Could you check a few things on this model? Use its own coordinates, in mm. A direction names the side the tool comes from. Coordinates: 2 decimals unless noted, no trailing zeros. Loops run counter-clockwise (first coordinate to the right, second up) from the corner with the lowest first, then second, coordinate; pieces in that order, holes last. Notation, with made-up numbers: (-4.5, -18.75) - (26.5, -18.75) arc R19 cw to (26.5, 0.25) - close; hole circle Ø4 at (43, 52). An arc over 180 degrees is marked (long way). One line per question, with ' | ' between items. Start each with the question number.
1. I want a section at A-A, the plane y = 3.25. Write out the boundary of the cut face in (x, z).
2. I want a section at B-B, the plane z = 0.15. Write out the boundary of the cut face in (x, y).
3. We'd pull the mould along X, two halves only. Please class faces 3 (the cylindrical face through (12.285, 0.301, 0.024)), 4 (the flat face through (18, 5, 0)), 5 (the flat face through (9, 6, -1.75)), 6 (the flat face through (0, 5, 0)): pulls with the +X half, pulls with the -X half, needs draft (parallel to the pull), parting line crosses it, or undercut.
4. Which directions (+Z, -Z, +X, -X, +Y, -Y) give clear straight access to the entire face, cutting with the end or side of a thin tool? Please do faces 1 (the cylindrical face through (17.43, 9.4, 0.02)), 2 (the cylindrical face through (5.699, 0.285, 0.024)).
5. I want a section at C-C, the plane x = 9. Write out the boundary of the cut face in (y, z).
6. Please list where these lines run through material, in increasing order: L1, parallel to X at y = 3.25, z = -0.7; L2, parallel to X at y = 4.25, z = 1.3; L3, parallel to X at y = 9, z = -0.1. Write a range as [from, to].
7. I want a section at D-D, the plane x = 11.25. Write out the boundary of the cut face in (y, z).
from build123d import *

# Parameters (mm, degrees)
BOSS_EXTRUDE1_DEPTH = 1.75


with BuildPart() as part:
    # Sketch1 → Boss-Extrude1 (new body, symmetric)
    with BuildSketch(Plane.XY):
        with BuildLine():
            Line((2, 0), (5, 0))
            ThreePointArc((5, 0), (5.707106781, 0.292893219), (6, 1))
            Line((6, 1), (6, 2))
            ThreePointArc((6, 2), (9, 5), (12, 2))
            Line((12, 2), (12, 1))
            ThreePointArc((12, 1), (12.292893219, 0.292893219), (13, 0))
            Line((13, 0), (16, 0))
            ThreePointArc((16, 0), (17.414213562, 0.585786438), (18, 2))
            Line((18, 2), (18, 8))
            ThreePointArc((18, 8), (17.414213562, 9.414213562), (16, 10))
            Line((16, 10), (2, 10))
            ThreePointArc((2, 10), (0.585786438, 9.414213562), (0, 8))
            Line((0, 8), (0, 2))
            ThreePointArc((0, 2), (0.585786438, 0.585786438), (2, 0))
        make_face()
    extrude(amount=BOSS_EXTRUDE1_DEPTH, both=True)


solid = part.part
Results are:
1) outline: (0, -1.75) - (6.27, -1.75) - (6.27, 1.75) - (0, 1.75) - close; (11.73, -1.75) - (18, -1.75) - (18, 1.75) - (11.73, 1.75) - close
2) outline: (0, 2) arc R2 ccw to (2, 0) - (5, 0) arc R1 ccw to (6, 1) - (6, 2) arc R3 cw to (12, 2) - (12, 1) arc R1 ccw to (13, 0) - (16, 0) arc R2 ccw to (18, 2) - (18, 8) arc R2 ccw to (16, 10) - (2, 10) arc R2 ccw to (0, 8) - close
3) face 3: undercut | face 4: pulls with the +X half | face 5: needs draft | face 6: pulls with the -X half
4) face 1: +Z, -Z, +X, +Y | face 2: +Z, -Z, -Y
5) outline: (5, -1.75) - (10, -1.75) - (10, 1.75) - (5, 1.75) - close
6) L1: x = [0, 6.27], [11.73, 18] | L2: x = [0, 7.02], [10.98, 18] | L3: x = [0.27, 17.73]
7) outline: (3.98, -1.75) - (10, -1.75) - (10, 1.75) - (3.98, 1.75) - close
